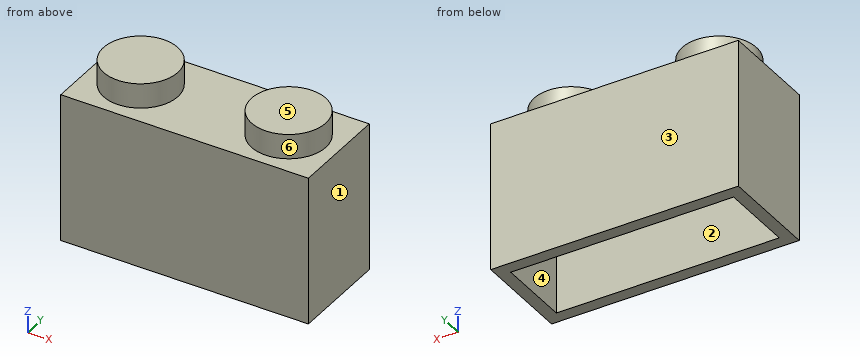
```python
from build123d import *

# Parameters (mm, degrees)
F0_W     = 100
F0_H     = 60
F1_DEPTH = 40
F3_R     = 15
F4_DEPTH = 10
F5_W     = 90
F5_H     = 30
F6_DEPTH = 40


with BuildPart() as f1:
    # F0 (on Front) → F1 (new body)
    with BuildSketch(Plane.XZ):
        Rectangle(F0_W, F0_H)
    extrude(amount=F1_DEPTH)

    # F3 (on face) → F4 (join)
    with BuildSketch(Plane.XY.offset(30)):
        with Locations((-30, -20)):
            Circle(F3_R)
        with Locations((30, -20.411897)):
            Circle(F3_R)
    extrude(amount=F4_DEPTH)

    # F5 (on face) → F6 (cut)
    with BuildSketch(Plane(origin=(0, 0, -30), x_dir=(1, 0, 0), z_dir=(0, 0, -1))):
        with Locations((0, 20)):
            Rectangle(F5_W, F5_H)
    extrude(amount=-F6_DEPTH, mode=Mode.SUBTRACT)


solid = f1.part
```
Geometry: final body of the model. Coordinates: model frame, mm. Face numbers are marked on the shaded views. A direction names the side the tool comes from. Give positions to 0.01 mm unless a question says otherwise; leave off trailing zeros. Write each loop counter-clockwise with the first axis right and the second up, starting at its lowest first coordinate (ties: lowest second). Pieces come first, ordered by that corner, then holes.
1. Draft query along X for the marked faces 1, 2 and 3. Return one class per face: released by +X, released by -X, zero draft, split by the parting line, or undercut.
2. Section query D-D, the plane x = -7. Return loops of the section in (y, z).
3. Line query: probe 1 along X at (y, z) = (-7.5, -4.5); probe 2 along Y at (x, z) = (22.5, -6); probe 3 along Z at (x, y) = (-12, -23.5). Output: solid intervals per line, ascending.
4. Reachability of the marked faces 4, 5 and 6 from +Z, -Z, +X, -X, +Y, -Y: full face, straight path, thin tool, end or side. Return the list, or none.
5. Pin query (flat end, axial travel): P1, Ø9, axis at x = -8, y = -15.5, coming from the -Z side. Return the tip coordinate at first contact, or that it passes through.
6. Section query B-B, the plane x = 30. Return loops of the section in (y, z), then the cut area to 3 significant figures.
7. Section query C-C, the plane y = -10.5. Return loops of the section in (x, z).
8. Section query A-A, the plane z = 3.5. Return loops of the section in (x, y).
Computed:
1. face 1: released by +X
1. face 2: undercut
1. face 3: zero draft
2. outline: (-40, -30) - (-35, -30) - (-35, 10) - (-5, 10) - (-5, -30) - (0, -30) - (0, 30) - (-40, 30) - close
3. probe 1: x = -50 to -45, 45 to 50
3. probe 2: y = -40 to -35, -5 to 0
3. probe 3: z = 10 to 30
4. face 4: -Z
4. face 5: +Z, +X, -X, +Y, -Y
4. face 6: +Z
5. P1: stops at z = 10
6. outline: (-40, -30) - (-35, -30) - (-35, 10) - (-5, 10) - (-5, -30) - (0, -30) - (0, 30) - (-5.41, 30) - (-5.41, 40) - (-35.41, 40) - (-35.41, 30) - (-40, 30) - close
6. area: 1,500 mm2
7. outline: (-50, -30) - (-45, -30) - (-45, 10) - (45, 10) - (45, -30) - (50, -30) - (50, 30) - (41.26, 30) - (41.26, 40) - (18.74, 40) - (18.74, 30) - (-18.39, 30) - (-18.39, 40) - (-41.61, 40) - (-41.61, 30) - (-50, 30) - close
8. outline: (-50, -40) - (50, -40) - (50, 0) - (-50, 0) - close; hole (-45, -35) - (45, -35) - (45, -5) - (-45, -5) - close
